from build123d import *

# Parameters (mm, degrees)
BOSS_EXTRUDE1_DEPTH = 6
BOSS_EXTRUDE2_START = 2
BOSS_EXTRUDE2_DEPTH = 2


with BuildPart() as part:
    # Sketch1 → Boss-Extrude1 (new, symmetric)
    with BuildSketch(Plane(origin=(0, 0, 0), x_dir=(1, 0, 0), z_dir=(0, 1, 0))):
        with BuildLine():
            Line((0, 0), (7, 0))
            ThreePointArc((7, 0), (7.875, -0.875), (7, -1.75))
            Line((7, -1.75), (0, -1.75))
            Line((0, -1.75), (0, -3.75))
            Line((0, -3.75), (5, -3.75))
            ThreePointArc((5, -3.75), (8.875, 0.125), (5, 4))
            Line((5, 4), (0, 4))
            Line((0, 4), (0, 0))
        make_face()
    extrude(amount=BOSS_EXTRUDE1_DEPTH, both=True)

    # Sketch2 → Boss-Extrude2 (add)
    with BuildSketch(Plane(origin=(0, 6, 0), x_dir=(1, 0, 0), z_dir=(0, 1, 0)).offset(BOSS_EXTRUDE2_START)):
        with BuildLine():
            Line((5, 6), (-2, 6))
            Line((-2, 6), (-2, 0))
            Line((-2, 0), (7, 0))
            ThreePointArc((7, 0), (7.875, -0.875), (7, -1.75))
            Line((7, -1.75), (-2, -1.75))
            Line((-2, -1.75), (-2, -5.75))
            Line((-2, -5.75), (5, -5.75))
            ThreePointArc((5, -5.75), (10.875, 0.125), (5, 6))
        make_face()
    boss_extrude2 = extrude(amount=-BOSS_EXTRUDE2_DEPTH)

    # Mirror1: Boss-Extrude2 across plane
    add(boss_extrude2.mirror(Plane.ZX))


solid = part.part
Geometry: final body of the model. Coordinates: model frame, mm. A direction names the side the tool comes from. Give positions to 0.01 mm unless a question says otherwise; leave off trailing zeros. Order: outer loops, then holes, each group sorted by start corner. A loop starts at its lowest first (then second) coordinate and runs counter-clockwise, first axis right, second up. Notation, with made-up numbers: (9, 10.25) -> (62, 10.25) arc R5 ccw to (62, 18.25) -> close; hole circle Ø5 at (-8, 12). An arc over 180 degrees is marked (long way). Answer as a JSON object with one key per item and string values.
Q1. Section D-D (z = -0.75). Output: boundary loops of the cut face in (x, y).
Entries:
{"outline": "(-2, -8) -> (10.84, -8) -> (10.84, -6) -> (8.82, -6) -> (8.82, 6) -> (10.84, 6) -> (10.84, 8) -> (-2, 8) -> (-2, 6) -> (0, 6) -> (0, -6) -> (-2, -6) -> close"}
Q2. Draft query along Z for faces 4 (the flat face through (1, -7, 5.75)), 5 (the cylindrical face through (7.875, -0.112, 0.856)), 6 (the flat face through (0, 0, -2)), 7 (the flat face through (2, -7, -6)). Return one class per face: released by +Z, released by -Z, zero draft, split by the parting line, or undercut.
Entries:
{"face 4": "released by +Z", "face 5": "undercut", "face 6": "zero draft", "face 7": "released by -Z"}
Q3. Section C-C (y = 0.5). Output: boundary loops of the cut face in (x, z) (3 decimals).
Entries:
{"outline": "(0, -4) -> (5, -4) arc R3.875 ccw to (5, 3.75) -> (0, 3.75) -> (0, 1.75) -> (7, 1.75) arc R0.875 cw to (7, 0) -> (0, 0) -> close"}
Q4. Section B-B (x = -0.25). Output: boundary loops of the cut face in (y, z).
Entries:
{"outline": "(-8, -6) -> (-6, -6) -> (-6, 0) -> (-8, 0) -> close; (-8, 1.75) -> (-6, 1.75) -> (-6, 5.75) -> (-8, 5.75) -> close; (6, -6) -> (8, -6) -> (8, 0) -> (6, 0) -> close; (6, 1.75) -> (8, 1.75) -> (8, 5.75) -> (6, 5.75) -> close"}
Q5. Material intervals for probe 1 along Z at (x, y) = (0.5, -1.25); probe 2 along Y at (x, z) = (9, -4); probe 3 along Z at (x, y) = (7.25, 2.5), sorted ascending.
Entries:
{"probe 1": "z = -4 to 0, 1.75 to 3.75", "probe 2": "y = -8 to -6, 6 to 8", "probe 3": "z = -3.28 to 0.04, 1.71 to 3.03"}
Q6. Access query for faces 1 (the flat face through (0, 0, 3)), 2 (the flat face through (5.8, -6, -4.1)), 3 (the flat face through (2, 0, 3.75)). Directions: +Z, -Z, +X, -X, +Y, -Y. A direction counts if a zero-diameter tool reaches every point of the face in a straight line with its end or side. Return the directions, or none.
Entries:
{"face 1": "+Z, -Z, -X", "face 2": "none", "face 3": "+Z, +X, -X"}
Q7. Section A-A (x = 4.75). Output: boundary loops of the cut face in (y, z).
Entries:
{"outline": "(-8, -6) -> (-6, -6) -> (-6, -4) -> (6, -4) -> (6, -6) -> (8, -6) -> (8, 0) -> (-8, 0) -> close; (-8, 1.75) -> (8, 1.75) -> (8, 5.75) -> (6, 5.75) -> (6, 3.75) -> (-6, 3.75) -> (-6, 5.75) -> (-8, 5.75) -> close"}
Q8. First-contact query: pin 1 (3 mm diameter, centred on y = 3.5, z = 2.5, fed in from +X); pin 2 (2 mm diameter, centred on y = 0.5, z = -3, fed in from -X); pin 3 (5.5 mm diameter, centred on x = 2, y = 0.5, fed in from +Z). Flat tips, straight axial feed; report the tip coordinate or a pass-through.
Entries:
{"pin 1": "stops at x = 8.71", "pin 2": "stops at x = 0", "pin 3": "stops at z = 3.75"}
